```python
from build123d import *

# Parameters (mm, degrees)
CHAMFER1_SIZE      = 1
M5_TAPPED_HOLE1_D  = 4.2
CUT_EXTRUDE1_DEPTH = 2.5
SKETCH6_W          = 1.15
SKETCH6_H          = 0.25


with BuildPart() as part:
    # Sketch1 → Revolve1 (revolve)
    with BuildSketch(Plane.XY):
        Polygon((0, 0), (0, 20), (7.5, 20), (7.5, 6), (103, 6), (103, 0), align=None)
    revolve(axis=Axis((103, 0, 0), (-1, 0, 0)))

    # Chamfer1
    chamfer1_edges = [part.edges().sort_by_distance(p)[0] for p in [
        (103, -6, 0),
        (7.5, -6, 0),
        (7.5, -20, 0),
        (0, -20, 0),
    ]]
    chamfer(chamfer1_edges, length=CHAMFER1_SIZE)

    # M5 Tapped Hole1 (through all)
    with Locations(Plane.ZY):
        with Locations((-12.5, 0), (0, 12.5), (12.5, 0), (0, -12.5)):
            Hole(M5_TAPPED_HOLE1_D / 2)

    # Sketch5 → Cut-Extrude1 (cut)
    with BuildSketch(Plane(origin=(0, 6, 0), x_dir=(1, 0, 0), z_dir=(0, 1, 0))):
        with BuildLine():
            Line((42.5, 2.5), (67.5, 2.5))
            ThreePointArc((67.5, 2.5), (70, 0), (67.5, -2.5))
            Line((67.5, -2.5), (42.5, -2.5))
            ThreePointArc((42.5, -2.5), (40, 0), (42.5, 2.5))
        make_face()
    extrude(amount=-CUT_EXTRUDE1_DEPTH, mode=Mode.SUBTRACT)

    # Sketch6 → Cut-Revolve1 (revolve, cut)
    with BuildSketch(Plane(origin=(0, 0, 0), x_dir=(1, 0, 0), z_dir=(0, 1, 0))):
        with Locations((100.425, 5.875)):
            Rectangle(SKETCH6_W, SKETCH6_H)
    revolve(axis=Axis((0, 0, 0), (1, 0, 0)), mode=Mode.SUBTRACT)


solid = part.part
```
Here's how the part is built. I have some questions about the finished solid (model axes, mm). A direction names the side the tool comes from. Coordinates: 2 decimals unless noted, no trailing zeros. Order: outer loops, then holes, each group sorted by start corner. A loop starts at its lowest first (then second) coordinate and runs counter-clockwise, first axis right, second up.
1) Will these pins go through, and if not, where does the flat tip stop? pin 1 (4 mm diameter, centred on x = 48, z = -1, fed in from +Y); pin 2 (2 mm diameter, centred on x = 59, y = 5, fed in from -Z); pin 3 (10 mm diameter, centred on y = 1, z = -12, fed in from +X); pin 4 (19 mm diameter, centred on y = 7, z = 8.5, fed in from +X).
2) Imagine slicing it at A-A on y = 0. State how many separate pieces and enclosed holes the cut face has, and give its area (3 significant figures).
3) Which directions (+Z, -Z, +X, -X, +Y, -Y) give clear straight access to the entire face, cutting with the end or side of a thin tool? Please do faces 1 (the face through (100.43, 5.7, 0.75)), 2 (the face through (7.5, 0, 8)), 3 (the face through (70, 5, 0)).
4) Imagine slicing it at C-C on x = 35. List the corners of the cut face in (y, z) for me.
5) I need wall thicknesses on line 1 (Y direction, x = 5.25, z = 0); line 2 (X direction, y = 6.5, z = -6.5); line 3 (Y direction, x = 4.25, z = 12.5). Which ranges of each line are inside material? Lowest first, please.
6) We'd pull the mould along X, two halves only. Please class faces 4 (the face through (103, 0, 0)), 5 (the face through (101.51, 5.54, 2.3)), 6 (the face through (55, 4, -2.5)): +X half, -X half, draft (parallel to the pull), parting line (faces both ways), or undercut.
Response values:
1. pin 1: stops at y = 5.45
1. pin 2: stops at z = -4.47
1. pin 3: stops at x = 7.5
1. pin 4: stops at x = 103
2. separate pieces: 3
2. enclosed holes: 0
2. area: 1,380 mm2
3. face 1: none
3. face 2: +X
3. face 3: +Y
4. outline: circle Ø12 at (0, 0)
5. line 1: y = -20 to -14.6, -10.4 to 10.4, 14.6 to 20
5. line 2: x = 0 to 7.5
5. line 3: y = -15.61 to -2.1, 2.1 to 15.61
6. face 4: +X half
6. face 5: draft
6. face 6: undercut
